```python
from build123d import *

# Parameters (mm, degrees)
CHAMFER1_SIZE = 0.2
CHAMFER2_SIZE = 0.2
CHAMFER3_SIZE = 0.2
CHAMFER4_SIZE = 0.2


with BuildPart() as part:
    # Sketch1 → Revolve1 (revolve)
    with BuildSketch(Plane(origin=(0, 0, 0), x_dir=(1, 0, 0), z_dir=(0, 1, 0))):
        with BuildLine():
            Line((2.75, 3.424799903), (2.75, 4))
            Line((2.75, 4), (2, 4))
            Line((2, 4), (2, 0))
            Line((2, 0), (2.75, 0))
            Line((2.75, 0), (2.75, 0.575200097))
            ThreePointArc((2.75, 0.575200097), (3.5, 0.25), (4.25, 0.575200097))
            Line((4.25, 0.575200097), (4.25, 0))
            Line((4.25, 0), (5, 0))
            Line((5, 0), (5, 4))
            Line((5, 4), (4.25, 4))
            Line((4.25, 4), (4.25, 3.424799903))
            ThreePointArc((4.25, 3.424799903), (3.5, 3.75), (2.75, 3.424799903))
        make_face()
    revolve(axis=Axis((0, 0, -4), (0, 0, 1)))

    # Chamfer1
    chamfer1_edges = [part.edges().sort_by_distance(p)[0] for p in [
        (-5, 0, -4),
    ]]
    chamfer(chamfer1_edges, length=CHAMFER1_SIZE)

    # Chamfer2
    chamfer2_edges = [part.edges().sort_by_distance(p)[0] for p in [
        (-2, 0, -4),
    ]]
    chamfer(chamfer2_edges, length=CHAMFER2_SIZE)

    # Chamfer3
    chamfer3_edges = [part.edges().sort_by_distance(p)[0] for p in [
        (-5, 0, 0),
    ]]
    chamfer(chamfer3_edges, length=CHAMFER3_SIZE)

    # Chamfer4
    chamfer4_edges = [part.edges().sort_by_distance(p)[0] for p in [
        (-2, 0, 0),
    ]]
    chamfer(chamfer4_edges, length=CHAMFER4_SIZE)


solid = part.part
```
Model file for the job. Use its own axes, mm. Coordinates: 2 decimals unless noted, no trailing zeros. Order: outer loops, then holes, each group sorted by start corner. A loop starts at its lowest first (then second) coordinate and runs counter-clockwise, first axis right, second up. Notation, with made-up numbers: (33, 36.25) -> (74, 36.25) arc R8 ccw to (74, 42.25) -> close; hole circle Ø4 at (-22.75, 61.25). An arc over 180 degrees is marked (long way). Return JSON: item names as keys, results as strings.
Item 1: Pin check, flat tips, straight feed: P1, Ø3, axis at x = 0, y = 0, coming from the +Z side; P2, Ø2, axis at y = -2, z = -2, coming from the +X side. Stop position of each tip, or through.
Model answer:
{"P1": "passes through", "P2": "stops at x = 4.9"}
Item 2: Slice it at C-C (z = -2). Write the cut outline in (x, y).
Model answer:
{"outline": "circle Ø10 at (0, 0); hole circle Ø4 at (0, 0)"}
Item 3: Mould opens along X. For faces 1 (the face through (2, -4, 0)), 2 (the face through (-1.08, -4.88, -2.03)), 3 (the face through (-0.596, -2.685, -0.292)) say: pulls with the +X half, pulls with the -X half, needs draft (parallel to the pull), parting line crosses it, or undercut.
Model answer:
{"face 1": "needs draft", "face 2": "parting line crosses it", "face 3": "undercut"}
Item 4: Slice it at D-D (z = -3.6). Write the cut outline in (x, y), then the cut area to 3 significant figures.
Model answer:
{"outline": "circle Ø10 at (0, 0); circle Ø8.07 at (0, 0); circle Ø5.5 at (0, 0); hole circle Ø8.5 at (0, 0); hole circle Ø5.93 at (0, 0); hole circle Ø4 at (0, 0)", "area": "56.5 mm²"}
Item 5: Wall check: line 1 along Y through (x, z) = (0, -1.45); line 2 along Y through (x, z) = (0, -0.4); line 3 along Y through (x, z) = (1.25, -2.15). Give the ranges that are in metal, low to high. Write a range as from..to.
Model answer:
{"line 1": "y = -5..-2, 2..5", "line 2": "y = -5..-4.25, -4.03..-2.97, -2.75..-2, 2..2.75, 2.97..4.03, 4.25..5", "line 3": "y = -4.84..-1.56, 1.56..4.84"}
